```python
from build123d import *

# Parameters (mm, degrees)
SKETCH_1_R      = 33
EXTRUDE_1_DEPTH = 70
SKETCH_2_W      = 16.190565304
SKETCH_2_H      = 61.081912216
EXTRUDE_3_DEPTH = 80


with BuildPart() as part:
    # 草图1 → 凸台-拉伸1 (new body)
    with BuildSketch(Plane.XY):
        Circle(SKETCH_1_R)
    extrude(amount=EXTRUDE_1_DEPTH)

    # 草图2 → 凸台-拉伸3 (add)
    with BuildSketch(Plane(origin=(0, 0, 0), x_dir=(-1, 0, 0), z_dir=(0, 0, -1))):
        with Locations((-20.595282652, 0)):
            Rectangle(SKETCH_2_W, SKETCH_2_H)
        with Locations((20.595282652, 0)):
            Rectangle(SKETCH_2_W, SKETCH_2_H)
    extrude(amount=EXTRUDE_3_DEPTH)


solid = part.part
```
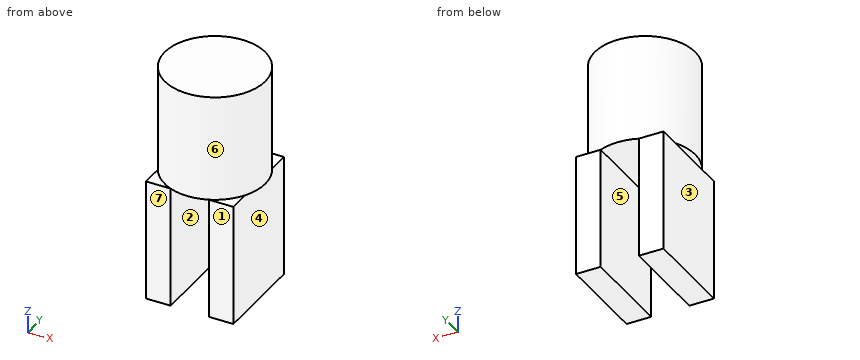
Geometry check sheet. Reference: the model listing, model coordinates, mm. Face numbers are marked on the shaded views. A direction names the side the tool comes from. Round coordinates to 2 decimals unless told otherwise and drop trailing zeros. Write each loop counter-clockwise with the first axis right and the second up, starting at its lowest first coordinate (ties: lowest second). Pieces come first, ordered by that corner, then holes. Notation, with made-up numbers: (-38.5, 57.25) - (-11.5, 57.25) arc R25 ccw to (-11.5, 92.25) - close; hole circle Ø5 at (61.25, 32.5). An arc over 180 degrees is marked (long way). Write each question's results on one line, items separated by ' | '.
(1) Sectioned sample at C-C, the plane x = -15. Enter the section's corners in (y, z), plus the area to 3 significant figures.
Computed:
outline: (-30.54, -80) - (30.54, -80) - (30.54, 0) - (29.39, 0) - (29.39, 70) - (-29.39, 70) - (-29.39, 0) - (-30.54, 0) - close | area: 9,000 mm^2
(2) Sectioned sample at A-A, the plane z = -43.5. Enter the section's corners in (x, y).
Computed:
outline: (-28.69, -30.54) - (-12.5, -30.54) - (-12.5, 30.54) - (-28.69, 30.54) - close; (12.5, -30.54) - (28.69, -30.54) - (28.69, 30.54) - (12.5, 30.54) - close
(3) Sectioned sample at D-D, the plane z = 10. Enter the section's corners in (x, y), plus the area to 3 significant figures.
Computed:
outline: circle Ø66 at (0, 0) | area: 3,420 mm^2
(4) Sectioned sample at B-B, the plane y = 0. Enter the section's corners in (x, z).
Computed:
outline: (-33, 0) - (-28.69, 0) - (-28.69, -80) - (-12.5, -80) - (-12.5, 0) - (12.5, 0) - (12.5, -80) - (28.69, -80) - (28.69, 0) - (33, 0) - (33, 70) - (-33, 70) - close
(5) Depth check by flat-ended pin: pin 1 Ø5 at (x, z) = (22.5, -48.5) entering from +Y; pin 2 Ø18 at (x, z) = (-24, -53) entering from -Y; pin 3 Ø7.5 at (x, y) = (-3.5, 3.5) entering from -Z; pin 4 Ø4.5 at (x, y) = (-30.5, 0.5) entering from -Z. Enter the tip coordinate at first touch or a pass-through.
Computed:
pin 1: stops at y = 30.54 | pin 2: stops at y = -30.54 | pin 3: stops at z = 0 | pin 4: stops at z = -80
(6) Set-up check for the marked faces 4, 5, 6 and 7: record each of +Z, -Z, +X, -X, +Y, -Y from which the full face is reachable in a straight line by a thin tool's end or side.
Computed:
face 4: -Z, +X, +Y, -Y | face 5: -Z, +Y, -Y | face 6: +Z | face 7: +Z, -Z, +X, -X, -Y
(7) Thickness scan on probe 1 along X at (y, z) = (-15, -44); probe 2 along Z at (x, y) = (-3, -16.5); probe 3 along Y at (x, z) = (17.5, -32). Record the ranges inside material, lowest first. Write a range as from..to.
Computed:
probe 1: x = -28.69..-12.5, 12.5..28.69 | probe 2: z = 0..70 | probe 3: y = -30.54..30.54
(8) Draft check along X on the marked faces 1, 2 and 3. Enter one of: pulls with the +X half, pulls with the -X half, needs draft (parallel to the pull), parting line crosses it, or undercut.
Computed:
face 1: needs draft | face 2: undercut | face 3: pulls with the -X half
